Design review of the part built by this model. Coordinates are the model's own, in mm. Give positions to 0.01 mm unless a question says otherwise; leave off trailing zeros. Order: outer loops, then holes, each group sorted by start corner. A loop starts at its lowest first (then second) coordinate and runs counter-clockwise, first axis right, second up.
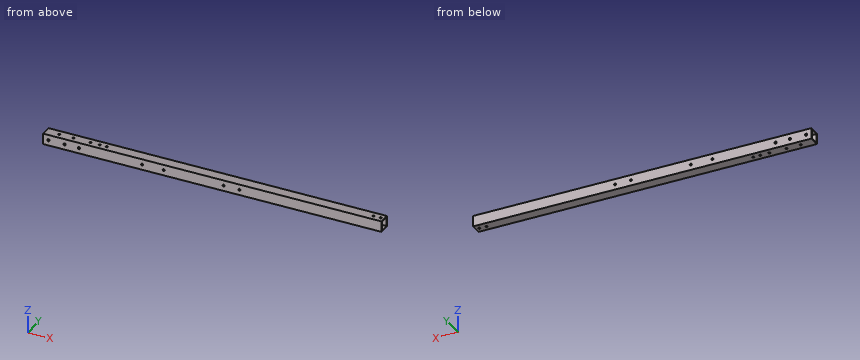
```python
from build123d import *

# Parameters (mm, degrees)
SKETCH_11_W         = 15
SKETCH_11_H         = 15
SKETCH_11_W_2       = 13
SKETCH_11_H_2       = 13
F_15X15X1_1_DEPTH   = 471
SKETCH_12_R         = 1.6
CUT_EXTRUDE_1_DEPTH = 237.096378625
SKETCH_13_R         = 1.45
CUT_EXTRUDE_2_DEPTH = 237.096378625
SKETCH_14_R         = 1.45
CUT_EXTRUDE_3_DEPTH = 237.096378625
SKETCH_15_R         = 1.45
CUT_EXTRUDE_4_DEPTH = 237.096378625
SKETCH_16_R         = 1.45
CUT_EXTRUDE_5_DEPTH = 237.096378625
SKETCH_18_R         = 1.45
CUT_EXTRUDE_7_DEPTH = 237.096378625


with BuildPart() as part:
    # 草图11 → 铝管 15X15X1(1) (new body)
    with BuildSketch(Plane(origin=(-235.5, 0, 0), x_dir=(0, 0, -1), z_dir=(1, 0, 0))):
        Rectangle(SKETCH_11_W, SKETCH_11_H)
        Rectangle(SKETCH_11_W_2, SKETCH_11_H_2, mode=Mode.SUBTRACT)
    extrude(amount=F_15X15X1_1_DEPTH)

    # 草图12 → 切除-拉伸1 (cut, through all)
    with BuildSketch(Plane(origin=(0, 7.5, 0), x_dir=(1, 0, 0), z_dir=(0, 1, 0))):
        with Locations(Location((-205.5, 0, 0), (0, 0, 270))):
            Circle(SKETCH_12_R)
        with Locations(Location((-185.5, 0, 0), (0, 0, 270))):
            Circle(SKETCH_12_R)
        with Locations(Location((-228, 0, 0), (0, 0, 270))):
            Circle(SKETCH_12_R)
    extrude(amount=-CUT_EXTRUDE_1_DEPTH, mode=Mode.SUBTRACT)

    # 草图13 → 切除-拉伸2 (cut, through all)
    with BuildSketch(Plane(origin=(0, 7.5, 0), x_dir=(1, 0, 0), z_dir=(0, 1, 0))):
        with Locations(Location((-97.5, 0, 0), (0, 0, 270))):
            Circle(SKETCH_13_R)
        with Locations(Location((-67.5, 0, 0), (0, 0, 270))):
            Circle(SKETCH_13_R)
    extrude(amount=-CUT_EXTRUDE_2_DEPTH, mode=Mode.SUBTRACT)

    # 草图14 → 切除-拉伸3 (cut, through all)
    with BuildSketch(Plane(origin=(0, 0, -7.5), x_dir=(-1, 0, 0), z_dir=(0, 0, -1))):
        with Locations((216.75, 0)):
            Circle(SKETCH_14_R)
        with Locations((196.75, 0)):
            Circle(SKETCH_14_R)
    extrude(amount=-CUT_EXTRUDE_3_DEPTH, mode=Mode.SUBTRACT)

    # 草图15 → 切除-拉伸4 (cut, through all)
    with BuildSketch(Plane(origin=(0, 0, -7.5), x_dir=(-1, 0, 0), z_dir=(0, 0, -1))):
        with Locations((173, 0)):
            Circle(SKETCH_15_R)
        with Locations((160.5, 0)):
            Circle(SKETCH_15_R)
        with Locations((150.5, 0)):
            Circle(SKETCH_15_R)
    extrude(amount=-CUT_EXTRUDE_4_DEPTH, mode=Mode.SUBTRACT)

    # 草图16 → 切除-拉伸5 (cut, through all)
    with BuildSketch(Plane(origin=(0, 0, -7.5), x_dir=(-1, 0, 0), z_dir=(0, 0, -1))):
        with Locations((-230.5, 0)):
            Circle(SKETCH_16_R)
        with Locations((-220.5, 0)):
            Circle(SKETCH_16_R)
    extrude(amount=-CUT_EXTRUDE_5_DEPTH, mode=Mode.SUBTRACT)

    # 草图18 → 切除-拉伸7 (cut, through all)
    with BuildSketch(Plane.XZ.offset(7.5)):
        with Locations(Location((15.7, 0, 0), (0, 0, 270))):
            Circle(SKETCH_18_R)
        with Locations(Location((37.7, 0, 0), (0, 0, 270))):
            Circle(SKETCH_18_R)
    extrude(amount=-CUT_EXTRUDE_7_DEPTH, mode=Mode.SUBTRACT)


solid = part.part
```
1. For line 1 along Z through (x, y) = (-174.5, 3.5); line 2 along Y through (x, z) = (-160.5, 7.2), list the stretches that pass through material, from the lowest coordinate up.
Recorded:
line 1: z = -7.5 to -6.5, 6.5 to 7.5
line 2: y = -7.5 to -1.45, 1.45 to 7.5
2. Take a section at A-A (y = -3.75). State the section outline as (x, z) points.
Recorded:
outline: (-235.5, -7.5) - (235.5, -7.5) - (235.5, -6.5) - (-235.5, -6.5) - close; (-235.5, 6.5) - (235.5, 6.5) - (235.5, 7.5) - (-235.5, 7.5) - close
3. For pin 1 (1.7 mm diameter, centred on x = 37.7, z = 0, fed in from -Y), flat-tipped, find the tip position at first contact; note if it passes through.
Recorded:
pin 1: passes through
4. Take a section at B-B (x = 103). State the section outline as (y, z) points, then the cut area to 3 significant figures.
Recorded:
outline: (-7.5, -7.5) - (7.5, -7.5) - (7.5, 7.5) - (-7.5, 7.5) - close; hole (-6.5, -6.5) - (6.5, -6.5) - (6.5, 6.5) - (-6.5, 6.5) - close
area: 56.0 mm2
